```python
from build123d import *

# Parameters (mm, degrees)
SKETCH1_R           = 5
BOSS_EXTRUDE1_DEPTH = 50


with BuildPart() as part:
    # Sketch1 → Boss-Extrude1 (new body)
    with BuildSketch(Plane(origin=(-24.036200878, 0, 0), x_dir=(0, 0, -1), z_dir=(1, 0, 0))):
        with BuildLine():
            ThreePointArc((-20.45966069, 14.943685115), (-19.408744482, 14.297932757), (-18.23009109, 13.93434348))
            ThreePointArc((-18.23009109, 13.93434348), (-18.241981361, 13.405873993), (-18.23009109, 12.877404505))
            ThreePointArc((-18.23009109, 12.877404505), (-19.408744482, 12.513815228), (-20.45966069, 11.86806287))
            ThreePointArc((-20.45966069, 11.86806287), (-20.423843041, 11.571709606), (-20.381738364, 11.276184046))
            ThreePointArc((-20.381738364, 11.276184046), (-19.19949825, 10.924432295), (-17.966902668, 10.878289967))
            ThreePointArc((-17.966902668, 10.878289967), (-17.84160982, 10.364750213), (-17.693346732, 9.857365315))
            ThreePointArc((-17.693346732, 9.857365315), (-18.737734654, 9.201107096), (-19.585708752, 8.305361087))
            ThreePointArc((-19.585708752, 8.305361087), (-19.465117023, 8.00599622), (-19.337681897, 7.709479816))
            ThreePointArc((-19.337681897, 7.709479816), (-18.111776725, 7.700053845), (-16.921717322, 7.994487129))
            ThreePointArc((-16.921717322, 7.994487129), (-16.667779856, 7.530873993), (-16.393247835, 7.079151127))
            ThreePointArc((-16.393247835, 7.079151127), (-17.232196976, 6.17494688), (-17.81944093, 5.09025083))
            ThreePointArc((-17.81944093, 5.09025083), (-17.640245305, 4.851510199), (-17.456018805, 4.616629895))
            ThreePointArc((-17.456018805, 4.616629895), (-16.256292957, 4.903124001), (-15.165762707, 5.479461363))
            ThreePointArc((-15.165762707, 5.479461363), (-14.80048604, 5.097369314), (-14.418393991, 4.732092647))
            ThreePointArc((-14.418393991, 4.732092647), (-14.994731353, 3.641562397), (-15.281225459, 2.441836549))
            ThreePointArc((-15.281225459, 2.441836549), (-15.046345155, 2.257610049), (-14.807604524, 2.078414424))
            ThreePointArc((-14.807604524, 2.078414424), (-13.722908474, 2.665658378), (-12.818704227, 3.504607519))
            ThreePointArc((-12.818704227, 3.504607519), (-12.366981361, 3.230075498), (-11.903368225, 2.976138032))
            ThreePointArc((-11.903368225, 2.976138032), (-12.17781737, 1.773599613), (-12.144037527, 0.540603301))
            ThreePointArc((-12.144037527, 0.540603301), (-11.869479248, 0.423445663), (-11.592494266, 0.312146602))
            ThreePointArc((-11.592494266, 0.312146602), (-10.696748258, 1.1601207), (-10.040490039, 2.204508622))
            ThreePointArc((-10.040490039, 2.204508622), (-9.533105141, 2.056245534), (-9.019565387, 1.930952686))
            ThreePointArc((-9.019565387, 1.930952686), (-8.973423058, 0.698357104), (-8.621671308, -0.48388301))
            ThreePointArc((-8.621671308, -0.48388301), (-8.326145748, -0.525987687), (-8.029792484, -0.561805336))
            ThreePointArc((-8.029792484, -0.561805336), (-7.384040126, 0.489110872), (-7.020450848, 1.667764264))
            ThreePointArc((-7.020450848, 1.667764264), (-6.491981361, 1.655873993), (-5.963511874, 1.667764264))
            ThreePointArc((-5.963511874, 1.667764264), (-5.599922596, 0.489110872), (-4.954170239, -0.561805336))
            ThreePointArc((-4.954170239, -0.561805336), (-4.657816975, -0.525987687), (-4.362291414, -0.48388301))
            ThreePointArc((-4.362291414, -0.48388301), (-4.010539664, 0.698357104), (-3.964397336, 1.930952686))
            ThreePointArc((-3.964397336, 1.930952686), (-3.450857581, 2.056245534), (-2.943472684, 2.204508622))
            ThreePointArc((-2.943472684, 2.204508622), (-2.287214465, 1.1601207), (-1.391468456, 0.312146602))
            ThreePointArc((-1.391468456, 0.312146602), (-1.114483475, 0.423445663), (-0.839925195, 0.540603301))
            ThreePointArc((-0.839925195, 0.540603301), (-0.806145353, 1.773599613), (-1.080594498, 2.976138032))
            ThreePointArc((-1.080594498, 2.976138032), (-0.616981361, 3.230075498), (-0.165258496, 3.504607519))
            ThreePointArc((-0.165258496, 3.504607519), (0.738945751, 2.665658378), (1.823641801, 2.078414424))
            ThreePointArc((1.823641801, 2.078414424), (2.062382432, 2.257610049), (2.297262736, 2.441836549))
            ThreePointArc((2.297262736, 2.441836549), (2.01076863, 3.641562397), (1.434431268, 4.732092647))
            ThreePointArc((1.434431268, 4.732092647), (1.816523318, 5.097369314), (2.181799984, 5.479461363))
            ThreePointArc((2.181799984, 5.479461363), (3.272330234, 4.903124001), (4.472056082, 4.616629895))
            ThreePointArc((4.472056082, 4.616629895), (4.656282582, 4.851510199), (4.835478208, 5.09025083))
            ThreePointArc((4.835478208, 5.09025083), (4.248234253, 6.17494688), (3.409285113, 7.079151127))
            ThreePointArc((3.409285113, 7.079151127), (3.683817133, 7.530873993), (3.9377546, 7.994487129))
            ThreePointArc((3.9377546, 7.994487129), (5.140293018, 7.720037984), (6.37328933, 7.753817827))
            ThreePointArc((6.37328933, 7.753817827), (6.490446969, 8.028376106), (6.601746029, 8.305361087))
            ThreePointArc((6.601746029, 8.305361087), (5.753771931, 9.201107096), (4.709384009, 9.857365315))
            ThreePointArc((4.709384009, 9.857365315), (4.857647098, 10.364750213), (4.982939945, 10.878289967))
            ThreePointArc((4.982939945, 10.878289967), (6.215535527, 10.924432295), (7.397775641, 11.276184046))
            ThreePointArc((7.397775641, 11.276184046), (7.439880319, 11.571709606), (7.475697967, 11.86806287))
            ThreePointArc((7.475697967, 11.86806287), (6.424781759, 12.513815228), (5.246128367, 12.877404505))
            ThreePointArc((5.246128367, 12.877404505), (5.258018639, 13.405873993), (5.246128367, 13.93434348))
            ThreePointArc((5.246128367, 13.93434348), (6.424781759, 14.297932757), (7.475697967, 14.943685115))
            ThreePointArc((7.475697967, 14.943685115), (7.439880319, 15.240038379), (7.397775641, 15.535563939))
            ThreePointArc((7.397775641, 15.535563939), (6.215535527, 15.88731569), (4.982939945, 15.933458018))
            ThreePointArc((4.982939945, 15.933458018), (4.857647098, 16.446997772), (4.709384009, 16.95438267))
            ThreePointArc((4.709384009, 16.95438267), (5.753771931, 17.610640889), (6.601746029, 18.506386898))
            ThreePointArc((6.601746029, 18.506386898), (6.490446969, 18.783371879), (6.37328933, 19.057930158))
            ThreePointArc((6.37328933, 19.057930158), (5.140293018, 19.091710001), (3.9377546, 18.817260856))
            ThreePointArc((3.9377546, 18.817260856), (3.683817133, 19.280873993), (3.409285113, 19.732596858))
            ThreePointArc((3.409285113, 19.732596858), (4.248234253, 20.636801105), (4.835478208, 21.721497155))
            ThreePointArc((4.835478208, 21.721497155), (4.656282582, 21.960237786), (4.472056082, 22.19511809))
            ThreePointArc((4.472056082, 22.19511809), (3.272330234, 21.908623984), (2.181799984, 21.332286622))
            ThreePointArc((2.181799984, 21.332286622), (1.816523318, 21.714378671), (1.434431268, 22.079655338))
            ThreePointArc((1.434431268, 22.079655338), (2.01076863, 23.170185588), (2.297262736, 24.369911436))
            ThreePointArc((2.297262736, 24.369911436), (2.062382432, 24.554137936), (1.823641801, 24.733333561))
            ThreePointArc((1.823641801, 24.733333561), (0.738945751, 24.146089607), (-0.165258496, 23.307140466))
            ThreePointArc((-0.165258496, 23.307140466), (-0.616981361, 23.581672487), (-1.080594498, 23.835609953))
            ThreePointArc((-1.080594498, 23.835609953), (-0.806145353, 25.038148372), (-0.839925195, 26.271144684))
            ThreePointArc((-0.839925195, 26.271144684), (-1.114483475, 26.388302322), (-1.391468456, 26.499601383))
            ThreePointArc((-1.391468456, 26.499601383), (-2.287214465, 25.651627285), (-2.943472684, 24.607239363))
            ThreePointArc((-2.943472684, 24.607239363), (-3.450857581, 24.755502451), (-3.964397336, 24.880795299))
            ThreePointArc((-3.964397336, 24.880795299), (-4.010539664, 26.113390881), (-4.362291414, 27.295630995))
            ThreePointArc((-4.362291414, 27.295630995), (-4.657816975, 27.337735672), (-4.954170239, 27.373553321))
            ThreePointArc((-4.954170239, 27.373553321), (-5.599922596, 26.322637113), (-5.963511874, 25.143983721))
            ThreePointArc((-5.963511874, 25.143983721), (-6.491981361, 25.155873993), (-7.020450848, 25.143983721))
            ThreePointArc((-7.020450848, 25.143983721), (-7.384040126, 26.322637113), (-8.029792484, 27.373553321))
            ThreePointArc((-8.029792484, 27.373553321), (-8.326145748, 27.337735672), (-8.621671308, 27.295630995))
            ThreePointArc((-8.621671308, 27.295630995), (-8.973423058, 26.113390881), (-9.019565387, 24.880795299))
            ThreePointArc((-9.019565387, 24.880795299), (-9.533105141, 24.755502451), (-10.040490039, 24.607239363))
            ThreePointArc((-10.040490039, 24.607239363), (-10.696748258, 25.651627285), (-11.592494266, 26.499601383))
            ThreePointArc((-11.592494266, 26.499601383), (-11.869479248, 26.388302322), (-12.144037527, 26.271144684))
            ThreePointArc((-12.144037527, 26.271144684), (-12.17781737, 25.038148372), (-11.903368225, 23.835609953))
            ThreePointArc((-11.903368225, 23.835609953), (-12.366981361, 23.581672487), (-12.818704227, 23.307140466))
            ThreePointArc((-12.818704227, 23.307140466), (-13.722908474, 24.146089607), (-14.807604524, 24.733333561))
            ThreePointArc((-14.807604524, 24.733333561), (-15.046345155, 24.554137936), (-15.281225459, 24.369911436))
            ThreePointArc((-15.281225459, 24.369911436), (-14.994731353, 23.170185588), (-14.418393991, 22.079655338))
            ThreePointArc((-14.418393991, 22.079655338), (-14.80048604, 21.714378671), (-15.165762707, 21.332286622))
            ThreePointArc((-15.165762707, 21.332286622), (-16.256292957, 21.908623984), (-17.456018805, 22.19511809))
            ThreePointArc((-17.456018805, 22.19511809), (-17.640245305, 21.960237786), (-17.81944093, 21.721497155))
            ThreePointArc((-17.81944093, 21.721497155), (-17.232196976, 20.636801105), (-16.393247835, 19.732596858))
            ThreePointArc((-16.393247835, 19.732596858), (-16.667779856, 19.280873993), (-16.921717322, 18.817260856))
            ThreePointArc((-16.921717322, 18.817260856), (-18.124255741, 19.091710001), (-19.357252053, 19.057930158))
            ThreePointArc((-19.357252053, 19.057930158), (-19.474409691, 18.783371879), (-19.585708752, 18.506386898))
            ThreePointArc((-19.585708752, 18.506386898), (-18.737734654, 17.610640889), (-17.693346732, 16.95438267))
            ThreePointArc((-17.693346732, 16.95438267), (-17.84160982, 16.446997772), (-17.966902668, 15.933458018))
            ThreePointArc((-17.966902668, 15.933458018), (-19.19949825, 15.88731569), (-20.381738364, 15.535563939))
            ThreePointArc((-20.381738364, 15.535563939), (-20.423843041, 15.240038379), (-20.45966069, 14.943685115))
        make_face()
        with Locations(Location((-6.491981361, 13.405873993, 0), (0, 0, 180))):
            Circle(SKETCH1_R, mode=Mode.SUBTRACT)
    extrude(amount=-BOSS_EXTRUDE1_DEPTH)


solid = part.part
```
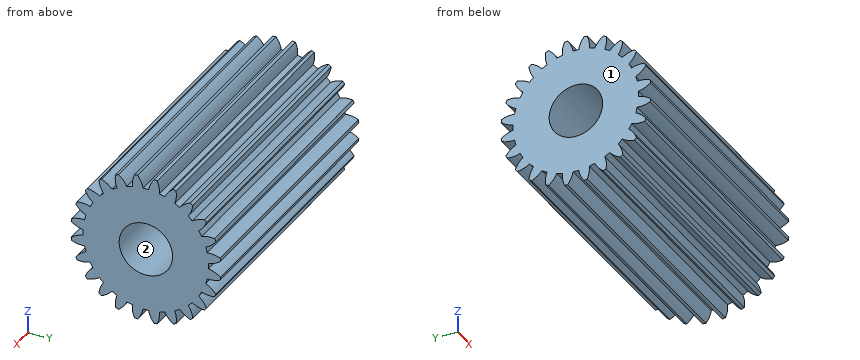
Geometry: final body of the model. Coordinates: model frame, mm. Face numbers are marked on the shaded views. Give positions to 0.01 mm unless a question says otherwise; leave off trailing zeros. Write each loop counter-clockwise with the first axis right and the second up, starting at its lowest first coordinate (ties: lowest second). Pieces come first, ordered by that corner, then holes.
1. Draft query along Z for the marked faces 1 and 2. Return one class per face: released by +Z, released by -Z, zero draft, split by the parting line, or undercut.
2. Section query B-B, the plane y = 20.75. Return loops of the section in (x, z), then the cut area to 3 significant figures.
3. Pin query (flat end, axial travel): P1, Ø2, axis at x = -52, y = 18.5, coming from the -Z side; P2, Ø8, axis at x = -41, z = -3, coming from the -Y side; P3, Ø1.5, axis at x = -41, y = 10, coming from the +Z side. Return the tip coordinate at first contact, or that it passes through.
4. Line query: probe 1 along Y at (x, z) = (-43.5, 6.5); probe 2 along Z at (x, y) = (-64.5, 25.75); probe 3 along Z at (x, y) = (-67.5, 3.25). Output: solid intervals per line, ascending.
5. Section query A-A, the plane y = 6. Return loops of the section in (x, z).
Computed:
1. face 1: zero draft
1. face 2: undercut
2. outline: (-74.04, -4.33) - (-24.04, -4.33) - (-24.04, 17.31) - (-74.04, 17.31) - close
2. area: 1,080 mm2
3. P1: stops at z = -6.6
3. P2: stops at y = 0.47
3. P3: stops at z = 18.68
4. probe 1: y = 1.66 to 8.41, 18.41 to 25.16
4. probe 2: z = 0.79 to 2.2, 3.96 to 5.82, 7.17 to 9.02, 10.78 to 12.2
4. probe 3: z = -2.14 to -0.06, 0.58 to 12.4, 13.05 to 15.12
5. outline: (-74.04, -4.37) - (-24.04, -4.37) - (-24.04, 17.35) - (-74.04, 17.35) - close
